Verification items for the finished model (mm, model axes). A direction names the side the tool comes from. Coordinates: 2 decimals unless noted, no trailing zeros. Loops run counter-clockwise (first coordinate to the right, second up) from the corner with the lowest first, then second, coordinate; pieces in that order, holes last. Notation, with made-up numbers: (-3.5, -31) -> (15.5, -31) arc R25 cw to (15.5, 2) -> close; hole circle Ø3 at (13, -38.75). An arc over 180 degrees is marked (long way). Use CSV: the item, a comma, the result in double quotes. Start each with the question number.
```python
from build123d import *

# Parameters (mm, degrees)
F0_R     = 2.5
F0_R_2   = 1.5
F1_DEPTH = 3


with BuildPart() as f1:
    # F0 (on Top) → F1 (new body)
    with BuildSketch(Plane.XY):
        with BuildLine():
            ThreePointArc((4.42411, -8.948789), (4.068757, -10.673534), (2.487618, -11.448789))
            Line((2.487618, -11.448789), (-1.258349, -11.448789))
            ThreePointArc((-1.258349, -11.448789), (-4.086776, -12.620362), (-5.258349, -15.448789))
            Line((-5.258349, -15.448789), (-5.258349, -54.828789))
            ThreePointArc((-5.258349, -54.828789), (-4.086776, -57.657216), (-1.258349, -58.828789))
            Line((-1.258349, -58.828789), (2.487618, -58.828789))
            ThreePointArc((2.487618, -58.828789), (4.068757, -59.604044), (4.42411, -61.328789))
            Line((4.42411, -61.328789), (4.709902, -106.048986))
            ThreePointArc((4.709902, -106.048986), (6.185581, -109.563846), (9.7098, -111.017033))
            Line((9.7098, -111.017033), (60.344679, -111.017033))
            ThreePointArc((60.344679, -111.017033), (63.891492, -109.541252), (65.344577, -105.985081))
            Line((65.344577, -105.985081), (65.059193, -61.328789))
            ThreePointArc((65.059193, -61.328789), (65.414546, -59.604044), (66.995685, -58.828789))
            Line((66.995685, -58.828789), (70.741651, -58.828789))
            ThreePointArc((70.741651, -58.828789), (73.570078, -57.657216), (74.741651, -54.828789))
            Line((74.741651, -54.828789), (74.741651, -15.448789))
            ThreePointArc((74.741651, -15.448789), (73.570078, -12.620362), (70.741651, -11.448789))
            Line((70.741651, -11.448789), (66.995685, -11.448789))
            ThreePointArc((66.995685, -11.448789), (65.414546, -10.673534), (65.059193, -8.948789))
            Line((65.059193, -8.948789), (65.059193, 18.551211))
            ThreePointArc((65.059193, 18.551211), (63.594727, 22.086745), (60.059193, 23.551211))
            Line((60.059193, 23.551211), (9.42411, 23.551211))
            ThreePointArc((9.42411, 23.551211), (5.888576, 22.086745), (4.42411, 18.551211))
            Line((4.42411, 18.551211), (4.42411, -8.948789))
        make_face()
        with Locations((-0.258349, -55.138789)):
            Circle(F0_R, mode=Mode.SUBTRACT)
        with BuildLine():
            ThreePointArc((10.741651, -74.638789), (11.327438, -73.224575), (12.741651, -72.638789))
            Line((12.741651, -72.638789), (56.741651, -72.638789))
            ThreePointArc((56.741651, -72.638789), (58.155865, -73.224575), (58.741651, -74.638789))
            Line((58.741651, -74.638789), (58.741651, -75.638789))
            ThreePointArc((58.741651, -75.638789), (58.155865, -77.053002), (56.741651, -77.638789))
            Line((56.741651, -77.638789), (12.741651, -77.638789))
            ThreePointArc((12.741651, -77.638789), (11.327438, -77.053002), (10.741651, -75.638789))
            Line((10.741651, -75.638789), (10.741651, -74.638789))
        make_face(mode=Mode.SUBTRACT)
        with BuildLine():
            Line((56.741651, -57.638789), (12.741651, -57.638789))
            ThreePointArc((12.741651, -57.638789), (11.327438, -57.053002), (10.741651, -55.638789))
            Line((10.741651, -55.638789), (10.741651, -54.638789))
            ThreePointArc((10.741651, -54.638789), (11.327438, -53.224575), (12.741651, -52.638789))
            Line((12.741651, -52.638789), (56.741651, -52.638789))
            ThreePointArc((56.741651, -52.638789), (58.155865, -53.224575), (58.741651, -54.638789))
            Line((58.741651, -54.638789), (58.741651, -55.638789))
            ThreePointArc((58.741651, -55.638789), (58.155865, -57.053002), (56.741651, -57.638789))
        make_face(mode=Mode.SUBTRACT)
        with Locations((69.741651, -55.138789)):
            Circle(F0_R, mode=Mode.SUBTRACT)
        with Locations((-0.258349, -20.138789)):
            Circle(F0_R, mode=Mode.SUBTRACT)
        with Locations((16.241651, -20.448789)):
            Circle(F0_R_2, mode=Mode.SUBTRACT)
        with Locations((16.241651, 16.551211)):
            Circle(F0_R_2, mode=Mode.SUBTRACT)
        with BuildLine():
            Line((12.741651, -32.638789), (56.741651, -32.638789))
            ThreePointArc((56.741651, -32.638789), (58.155865, -33.224575), (58.741651, -34.638789))
            Line((58.741651, -34.638789), (58.741651, -35.638789))
            ThreePointArc((58.741651, -35.638789), (58.155865, -37.053002), (56.741651, -37.638789))
            Line((56.741651, -37.638789), (12.741651, -37.638789))
            ThreePointArc((12.741651, -37.638789), (11.327438, -37.053002), (10.741651, -35.638789))
            Line((10.741651, -35.638789), (10.741651, -34.638789))
            ThreePointArc((10.741651, -34.638789), (11.327438, -33.224575), (12.741651, -32.638789))
        make_face(mode=Mode.SUBTRACT)
        with Locations((53.241651, -20.448789)):
            Circle(F0_R_2, mode=Mode.SUBTRACT)
        with Locations((69.741651, -20.138789)):
            Circle(F0_R, mode=Mode.SUBTRACT)
        with BuildLine():
            Line((56.741651, 2.361211), (12.741651, 2.361211))
            ThreePointArc((12.741651, 2.361211), (11.327438, 2.946998), (10.741651, 4.361211))
            Line((10.741651, 4.361211), (10.741651, 5.361211))
            ThreePointArc((10.741651, 5.361211), (11.327438, 6.775425), (12.741651, 7.361211))
            Line((12.741651, 7.361211), (56.741651, 7.361211))
            ThreePointArc((56.741651, 7.361211), (58.155865, 6.775425), (58.741651, 5.361211))
            Line((58.741651, 5.361211), (58.741651, 4.361211))
            ThreePointArc((58.741651, 4.361211), (58.155865, 2.946998), (56.741651, 2.361211))
        make_face(mode=Mode.SUBTRACT)
        with Locations((53.241651, 16.551211)):
            Circle(F0_R_2, mode=Mode.SUBTRACT)
    extrude(amount=-F1_DEPTH)


solid = f1.part
```
1. Release check for a two-part mould opening along Y. For faces 1 (the flat face through (69, -11.449, -1)), 2 (the flat face through (4.424, 5, -1)), 3 (the cylindrical face through (52.05, -21.36, -1.48)) record: released by +Y, released by -Y, zero draft, split by the parting line, or undercut.
2. Set-up check for faces 4 (the flat face through (1, -11.449, -1)), 5 (the flat face through (34, -32.639, -1)), 6 (the flat face through (65.059, 5, -1)), 7 (the flat face through (1, -58.829, -1)): record each of +Z, -Z, +X, -X, +Y, -Y from which the full face is reachable in a straight line by a thin tool's end or side.
3. Scan lines: line 1 (Y direction, x = 13.5, z = -1.7); line 2 (X direction, y = 16.5, z = -0.3); line 3 (X direction, y = -34.5, z = -0.6). Record each from-to range of solid material in increasing order.
4. Cross-section at A-A, the plane x = 23.5. Record the boundary of the cut face in (y, z), plus the area to 3 significant figures.
5. Cross-section at B-B, the plane x = 53. Record the boundary of the cut face in (y, z), plus the area to 3 significant figures.
6. Depth check by flat-ended pin: pin 1 (2.5 mm diameter, centred on x = 16.24, y = 16.55, fed in from -Z). Enter the tip coordinate at first touch or a pass-through.
7. Cross-section at C-C, the plane z = -1.3. State how many separate pieces and enclosed holes the cut face has, plus the area to 3 significant figures.
8. Cross-section at D-D, the plane y = -89.5. Record the boundary of the cut face in (x, z).
Solution:
1,face 1,"released by +Y"
1,face 2,"zero draft"
1,face 3,"undercut"
2,face 4,"+Z, -Z, -X, +Y"
2,face 5,"+Z, -Z"
2,face 6,"+Z, -Z, +X, +Y"
2,face 7,"+Z, -Z, -X, -Y"
3,line 1,"y = -111.02 to -77.64, -72.64 to -57.64, -52.64 to -37.64, -32.64 to 2.36, 7.36 to 23.55"
3,line 2,"x = 4.42 to 14.74, 17.74 to 51.74, 54.74 to 65.06"
3,line 3,"x = -5.26 to 10.75, 58.74 to 74.74"
4,outline,"(-111.02, -3) -> (-77.64, -3) -> (-77.64, 0) -> (-111.02, 0) -> close; (-72.64, -3) -> (-57.64, -3) -> (-57.64, 0) -> (-72.64, 0) -> close; (-52.64, -3) -> (-37.64, -3) -> (-37.64, 0) -> (-52.64, 0) -> close; (-32.64, -3) -> (2.36, -3) -> (2.36, 0) -> (-32.64, 0) -> close; (7.36, -3) -> (23.55, -3) -> (23.55, 0) -> (7.36, 0) -> close"
4,area,"344 mm2"
5,outline,"(-111.02, -3) -> (-77.64, -3) -> (-77.64, 0) -> (-111.02, 0) -> close; (-72.64, -3) -> (-57.64, -3) -> (-57.64, 0) -> (-72.64, 0) -> close; (-52.64, -3) -> (-37.64, -3) -> (-37.64, 0) -> (-52.64, 0) -> close; (-32.64, -3) -> (-21.93, -3) -> (-21.93, 0) -> (-32.64, 0) -> close; (-18.97, -3) -> (2.36, -3) -> (2.36, 0) -> (-18.97, 0) -> close; (7.36, -3) -> (15.07, -3) -> (15.07, 0) -> (7.36, 0) -> close; (18.03, -3) -> (23.55, -3) -> (23.55, 0) -> (18.03, 0) -> close"
5,area,"326 mm2"
6,pin 1,"passes through"
7,separate pieces,"1"
7,enclosed holes,"12"
7,area,"7,990 mm2"
8,outline,"(4.6, -3) -> (65.24, -3) -> (65.24, 0) -> (4.6, 0) -> close"
